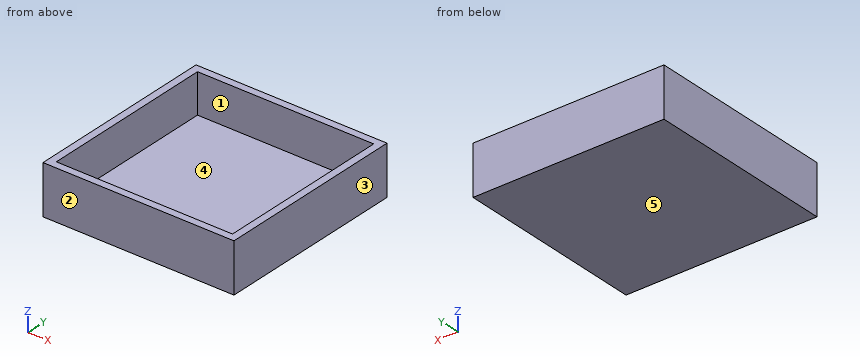
```python
from build123d import *

# Parameters (mm, degrees)
F0_W     = 155
F0_H     = 155
F1_DEPTH = 40
F2_T     = -6
F3_DEPTH = 2


with BuildPart() as f1:
    # F0 (on Top) → F1 (new body)
    with BuildSketch(Plane.XY):
        Rectangle(F0_W, F0_H)
    extrude(amount=F1_DEPTH)

    # F2
    f2_openings = [f1.faces().sort_by_distance(p)[0] for p in [
        (0, 0, 40),
    ]]
    offset(amount=F2_T, openings=f2_openings)

    # F3 (add): a face of the model
    f3_faces = [f1.faces().sort_by_distance(p)[0] for p in [
        (0, 0, 6),
    ]]
    extrude(f3_faces, amount=F3_DEPTH)


solid = f1.part
```
CAD build for the part. Positions are in the model's coordinates, mm. Face numbers are marked on the shaded views. A direction names the side the tool comes from. Round coordinates to 2 decimals unless told otherwise and drop trailing zeros. Loops run counter-clockwise (first coordinate to the right, second up) from the corner with the lowest first, then second, coordinate; pieces in that order, holes last. Notation, with made-up numbers: (-26.75, 44.25) - (-0.75, 44.25) arc R22 ccw to (-0.75, 65.25) - close; hole circle Ø1 at (-11.5, 65.25). An arc over 180 degrees is marked (long way). Return JSON: item names as keys, results as strings. Group by question number.
Q1. Two-plate mould, pull along X, no slides. Class the marked faces 3, 4 and 5: +X half, -X half, draft (parallel to the pull), parting line (faces both ways), or undercut.
Q2. Band-saw the part on B-B on x = 16. Give the cut face in (y, z), plus the area to 3 significant figures.
Q3. Band-saw the part on A-A on z = 37. Give the cut face in (x, y), plus the area to 3 significant figures.
Q4. Tool access for the marked faces 1 and 2: list every direction of +Z, -Z, +X, -X, +Y, -Y with a clear straight run to the whole face (end or side of a thin tool).
Q5. Drill centre lines: line 1 along X through (y, z) = (4, 29); line 2 along Z through (x, y) = (46.5, 64). Where is each one in solid material? Low to high. Write a range as [from, to].
Q6. Flat gauge pin, fed straight in: pin 1 Ø10 at (x, y) = (45, -28.5) entering from +Z. Where does the tip first touch, or does it go through?
Solutions:
{
 "1": {"face 3": "+X half", "face 4": "undercut", "face 5": "draft"},
 "2": {"outline": "(-77.5, 0) - (77.5, 0) - (77.5, 40) - (71.5, 40) - (71.5, 8) - (-71.5, 8) - (-71.5, 40) - (-77.5, 40) - close", "area": "1,620 mm^2"},
 "3": {"outline": "(-77.5, -77.5) - (77.5, -77.5) - (77.5, 77.5) - (-77.5, 77.5) - close; hole (-71.5, -71.5) - (71.5, -71.5) - (71.5, 71.5) - (-71.5, 71.5) - close", "area": "3,580 mm^2"},
 "4": {"face 1": "+Z", "face 2": "+Z, -Z, +X, -X, -Y"},
 "5": {"line 1": "x = [-77.5, -71.5], [71.5, 77.5]", "line 2": "z = [0, 8]"},
 "6": {"pin 1": "stops at z = 8"}
}
